Check sheet for the drawn part. Datum: minimum x, y, z corner. Units: mm. Give positions to 0.01 mm unless a question says otherwise; leave off trailing zeros. Write each loop counter-clockwise with the first axis right and the second up, starting at its lowest first coordinate (ties: lowest second). Pieces come first, ordered by that corner, then holes. Notation, with made-up numbers: (21.25, -29) -> (64.25, -29) arc R21 ccw to (64.25, 7) -> close; hole circle Ø6 at (61.25, -25.75). An arc over 180 degrees is marked (long way). Write item = value, one per line. Start each with the question number.
1. Cross-section at C-C, the plane x = 10. Record the cut outline in (y, z).
2. Cross-section at D-D, the plane z = 22. Record the cut outline in (x, y).
3. Mould release check, pull along X, two halves, no side actions. Record for the marked faces 1, 2, 3 and 4: pulls with the +X half, pulls with the -X half, needs draft (parallel to the pull), parting line crosses it, or undercut.
4. Depth check by flat-ended pin: P1, Ø2, axis at x = 17, y = 8, coming from the +Z side. Enter the tip coordinate at first touch or a pass-through.
5. Cross-section at A-A, the plane z = 12.5. Record the cut outline in (x, y), plus the area to 3 significant figures.
6. Cross-section at B-B, the plane y = 4. Record the cut outline in (x, z), plus the area to 3 significant figures.
7. Thickness scan on line 1 along X through (y, z) = (4.75, 14.75); line 2 along Z through (x, y) = (10, 3.75); line 3 along X through (y, z) = (5.25, 19.25). Record the ranges inside material, lowest first.
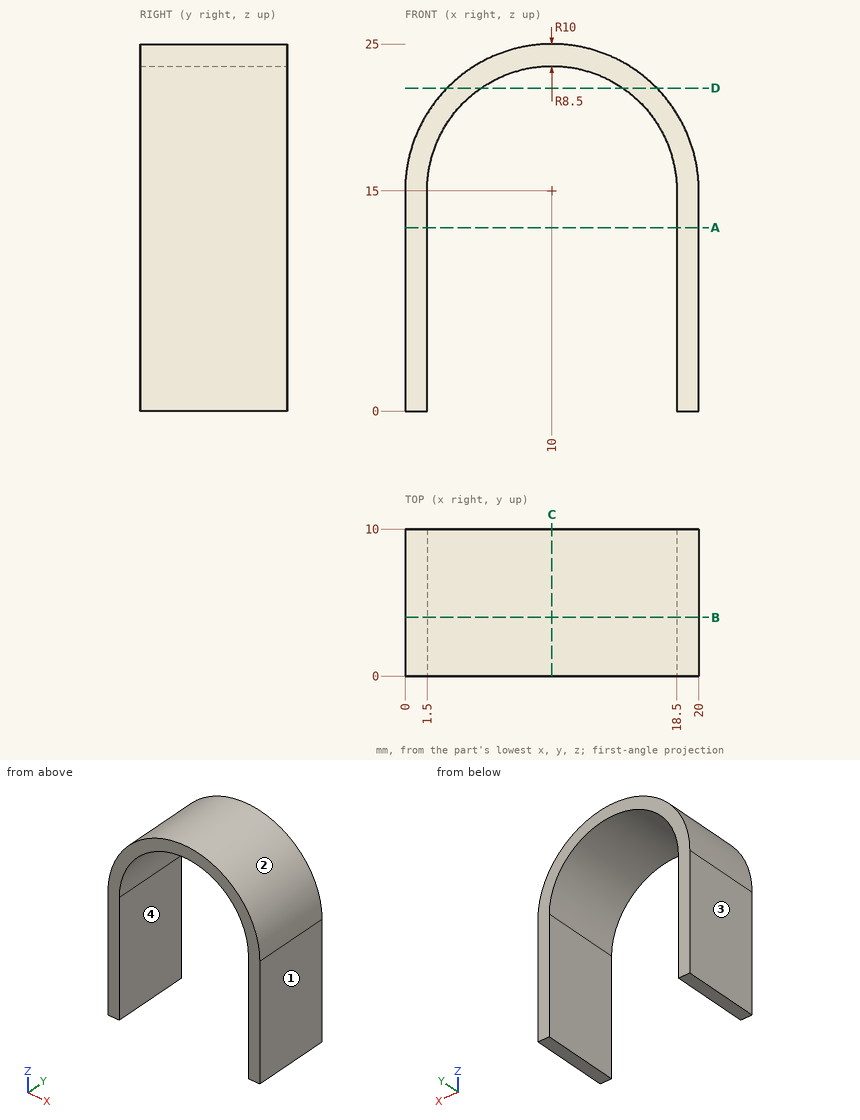
Answers:
q1.outline = (0, 23.5) -> (10, 23.5) -> (10, 25) -> (0, 25) -> close
q2.outline = (2.86, 0) -> (5.18, 0) -> (5.18, 10) -> (2.86, 10) -> close; (14.82, 0) -> (17.14, 0) -> (17.14, 10) -> (14.82, 10) -> close
q3.face_1 = pulls with the +X half
q3.face_2 = parting line crosses it
q3.face_3 = pulls with the -X half
q3.face_4 = undercut
q4.P1 = 23
q5.outline = (0, 0) -> (1.5, 0) -> (1.5, 10) -> (0, 10) -> close; (18.5, 0) -> (20, 0) -> (20, 10) -> (18.5, 10) -> close
q5.area = 30.0 mm^2
q6.outline = (0, 0) -> (1.5, 0) -> (1.5, 15) arc R8.5 cw to (18.5, 15) -> (18.5, 0) -> (20, 0) -> (20, 15) arc R10 ccw to (0, 15) -> close
q6.area = 88.6 mm^2
q7.line_1 = 0 to 1.5, 18.5 to 20
q7.line_2 = 23.5 to 25
q7.line_3 = 0.95 to 2.64, 17.36 to 19.05
